The model under review builds one solid part; all positions refer to its coordinate system, in mm. A direction names the side the tool comes from. Round coordinates to 2 decimals unless told otherwise and drop trailing zeros. Order: outer loops, then holes, each group sorted by start corner. A loop starts at its lowest first (then second) coordinate and runs counter-clockwise, first axis right, second up. Notation, with made-up numbers: (-19, -8) -> (7, -8) arc R13 ccw to (7, 6) -> close; hole circle Ø3 at (21.5, 86). An arc over 180 degrees is marked (long way). Put each result on its own line as item: value. Start each with the question number.
from build123d import *

# Parameters (mm, degrees)
SKETCH1_W                 = 340
SKETCH1_H                 = 150
VERTICAL_PORTION_DEPTH    = 10
SHAFT_ADAPTER_RIGHT_DEPTH = 25
SHAFT_ADAPTER_FILLETS_R   = 5


with BuildPart() as part:
    # Sketch1 → Vertical portion (new body)
    with BuildSketch(Plane.XY):
        Rectangle(SKETCH1_W, SKETCH1_H)
    extrude(amount=VERTICAL_PORTION_DEPTH)

    # Sketch4 → Shaft adapter right (add)
    with BuildSketch(Plane(origin=(155, 0, 0), x_dir=(0, 0, -1), z_dir=(1, 0, 0))):
        with BuildLine():
            Line((-10, 45), (-30, 52.5))
            Line((-30, 52.5), (-30, 60))
            Line((-30, 60), (-25, 60))
            ThreePointArc((-25, 60), (-20, 55), (-15, 60))
            Line((-15, 60), (-10, 60))
            Line((-10, 60), (-10, 55))
            Line((-10, 55), (-10, 45))
        make_face()
    shaft_adapter_right = extrude(amount=-SHAFT_ADAPTER_RIGHT_DEPTH)

    # Shaft adapter left: Shaft adapter right across plane
    add(shaft_adapter_right.mirror(Plane(origin=(0, 0, 0), x_dir=(0, 0, 1), z_dir=(1, 0, 0))))

    # Shaft adapter fillets
    shaft_adapter_fillets_edges = [part.edges().sort_by_distance(p)[0] for p in [
        (-142.5, 52.5, 30),
        (142.5, 52.5, 30),
        (130, 52.5, 10),
        (-130, 52.5, 10),
        (-142.5, 45, 10),
        (142.5, 45, 10),
        (142.5, 60, 10),
        (-142.5, 60, 10),
    ]]
    fillet(shaft_adapter_fillets_edges, radius=SHAFT_ADAPTER_FILLETS_R - 0.0001)  # a hair under: the kernel refuses the full size


solid = part.part
Q1. Take a section at B-B on x = 38.5. Give the boundary of the cut face in (y, z), and give its area (3 significant figures).
Q2. Take a section at A-A on z = 20. Give the boundary of the cut face in (x, y), and give its area (4 significant figures).
Q3. Wall thickness on probe 1 along Z at (x, y) = (80.5, 34.5); probe 2 along Y at (x, z) = (-153, 26.75); probe 3 along Y at (x, z) = (-138, 23) (3 decimals): over which ranges is each line inside the solid? List them lowest first. Write a range as [from, to].
Q4. Clearance check with flat-ended pins moving along their axes: pin 1 Ø4 at (x, z) = (143, 27) entering from +Y; pin 2 Ø10.5 at (y, z) = (53, 21.5) entering from +X; pin 3 Ø5 at (y, z) = (14, 13.5) entering from -X (1 decimal); pin 4 Ø10 at (y, z) = (50, 18.5) entering from -X. State where each tip first meets the part, or that it passes through.
Q5. Take a section at C-C on y = -60.5. Give the boundary of the cut face in (x, z), and give its area (3 significant figures).
Q6. Draft analysis for pull direction X (two halves, no side actions). For faces 3 (the face through (-2, -75, 5)), 4 (the face through (155, 53, 18)), 5 (the face through (130, 54, 22)), 6 (the face through (-155, 53, 18)), state which applies: +X half, -X half, draft (parallel to the pull), parting line (faces both ways), or undercut.
Q7. For faces 1 (the face through (170, -1, 5)), 2 (the face through (-130, 54, 22)), list the 3-axis set-ups (+Z, -Z, +X, -X, +Y, -Y) from which the entire face can be reached by the end or side of a thin tool; tool diameter is ignored.
Calculated:
1. outline: (-75, 0) -> (75, 0) -> (75, 10) -> (-75, 10) -> close
1. area: 1,500 mm²
2. outline: (-155, 48.75) -> (-130, 48.75) -> (-130, 55) -> (-155, 55) -> close; (130, 48.75) -> (155, 48.75) -> (155, 55) -> (130, 55) -> close
2. area: 312.5 mm²
3. probe 1: z = [0, 10]
3. probe 2: y = [51.28, 60]
3. probe 3: y = [49.875, 56]
4. pin 1: stops at y = 60
4. pin 2: stops at x = 155
4. pin 3: passes through
4. pin 4: stops at x = -155
5. outline: (-170, 0) -> (170, 0) -> (170, 10) -> (-170, 10) -> close
5. area: 3,400 mm²
6. face 3: draft
6. face 4: +X half
6. face 5: undercut
6. face 6: -X half
7. face 1: +Z, -Z, +X, +Y, -Y
7. face 2: +Z, +Y, -Y
